Design review of the part built by this model. Coordinates are the model's own, in mm. Round coordinates to 2 decimals unless told otherwise and drop trailing zeros. Order: outer loops, then holes, each group sorted by start corner. A loop starts at its lowest first (then second) coordinate and runs counter-clockwise, first axis right, second up. Notation, with made-up numbers: M -39.5,59.5 L -24.5,59.5 A24 cw -24.5,78.5 Z; hole C 5,-12.5 d6. An arc over 180 degrees is marked long. Use a Markdown table: item, result. Add a question column.
(1) Take a section at A-A (z = 0.35). Count the separate pieces of the cut face and the enclosed holes in it, then the cut area to 3 significant figures.
(2) To check wall thickness, follow probe 1 along Y at (x, z) = (8, 1.1); probe 2 along X at (y, z) = (-3.75, 0.7); probe 3 along X at (y, z) = (-3.25, 1.15). State the ranges of each line that lie inside material, in increasing order. Write a range as from..to.
(3) The part is to be moulded in two halves that separate along X. For faces 1 (the face through (9.76, -3.05, 0.79)), 2 (the face through (5, -5.08, 1)), 3 (the face through (1.524, 0, 1)), say which applies: released by +X, released by -X, zero draft, split by the parting line, or undercut.
(4) Take a section at B-B (x = 82.55). Write out the cut boundary in (y, z), then the cut area to 3 significant figures.
(5) For pin 1 (1.5 mm diameter, centred on x = 25, y = -3, fed in from -Z), flat-tipped, find the tip position at first contact; note if it passes through.
```python
from build123d import *

# Parameters (mm, degrees)
SKETCH_2_R      = 0.325658607
EXTRUDE_1_DEPTH = 1.6


with BuildPart() as part:
    # 草图2 → 凸台-拉伸1 (new body)
    with BuildSketch(Plane.XY):
        with BuildLine():
            Line((1.524, 5.08), (1.524, -5.08))
            Line((1.524, -5.08), (8.763, -5.08))
            Line((8.763, -5.08), (8.763, -4.064))
            ThreePointArc((8.763, -4.064), (9.779, -3.048), (10.795, -4.064))
            Line((10.795, -4.064), (10.795, -5.08))
            Line((10.795, -5.08), (81.534, -5.08))
            Line((81.534, -5.08), (81.534, -4.064))
            ThreePointArc((81.534, -4.064), (82.55, -3.048), (83.566, -4.064))
            Line((83.566, -4.064), (83.566, -5.08))
            Line((83.566, -5.08), (91.059, -5.08))
            Line((91.059, -5.08), (91.059, 5.08))
            Line((91.059, 5.08), (83.566, 5.08))
            Line((83.566, 5.08), (83.566, 4.064))
            ThreePointArc((83.566, 4.064), (82.55, 3.048), (81.534, 4.064))
            Line((81.534, 4.064), (81.534, 5.08))
            Line((81.534, 5.08), (10.795, 5.08))
            Line((10.795, 5.08), (10.795, 4.064))
            ThreePointArc((10.795, 4.064), (9.779, 3.048), (8.763, 4.064))
            Line((8.763, 4.064), (8.763, 5.08))
            Line((8.763, 5.08), (1.524, 5.08))
        make_face()
        with Locations((6.937038713, 2.89)):
            Circle(SKETCH_2_R, mode=Mode.SUBTRACT)
        with Locations((6.937038713, -2.89)):
            Circle(SKETCH_2_R, mode=Mode.SUBTRACT)
        with BuildLine():
            Line((2.982, 4.62), (3.602, 4.62))
            ThreePointArc((3.602, 4.62), (3.902, 4.32), (3.602, 4.02))
            Line((3.602, 4.02), (2.982, 4.02))
            ThreePointArc((2.982, 4.02), (2.682, 4.32), (2.982, 4.62))
        make_face(mode=Mode.SUBTRACT)
        with BuildLine():
            Line((6.917, 4.62), (8.017, 4.62))
            ThreePointArc((8.017, 4.62), (8.317, 4.32), (8.017, 4.02))
            Line((8.017, 4.02), (6.917, 4.02))
            ThreePointArc((6.917, 4.02), (6.617, 4.32), (6.917, 4.62))
        make_face(mode=Mode.SUBTRACT)
        with BuildLine():
            Line((8.017, -4.02), (6.917, -4.02))
            ThreePointArc((6.917, -4.02), (6.617, -4.32), (6.917, -4.62))
            Line((6.917, -4.62), (8.017, -4.62))
            ThreePointArc((8.017, -4.62), (8.317, -4.32), (8.017, -4.02))
        make_face(mode=Mode.SUBTRACT)
        with BuildLine():
            Line((3.602, -4.02), (2.982, -4.02))
            ThreePointArc((2.982, -4.02), (2.682, -4.32), (2.982, -4.62))
            Line((2.982, -4.62), (3.602, -4.62))
            ThreePointArc((3.602, -4.62), (3.902, -4.32), (3.602, -4.02))
        make_face(mode=Mode.SUBTRACT)
    extrude(amount=EXTRUDE_1_DEPTH)


solid = part.part
```
Verdict:
| question | item | result |
|---|---|---|
| 1 | separate pieces | 1 |
| 1 | enclosed holes | 6 |
| 1 | area | 891 mm^2 |
| 2 | probe 1 | y = -5.08..-4.62, -4.02..4.02, 4.62..5.08 |
| 2 | probe 2 | x = 1.52..8.81, 10.75..81.58, 83.52..91.06 |
| 2 | probe 3 | x = 1.52..9.17, 10.39..81.94, 83.16..91.06 |
| 3 | face 1 | undercut |
| 3 | face 2 | zero draft |
| 3 | face 3 | released by -X |
| 4 | outline | M -3.05,0 L 3.05,0 L 3.05,1.6 L -3.05,1.6 Z |
| 4 | area | 9.75 mm^2 |
| 5 | pin 1 | stops at z = 0 |
